Can you work these out from the model? Positions are in its coordinate system, mm. Face numbers are marked on the shaded views. A direction names the side the tool comes from. Coordinates: 2 decimals unless noted, no trailing zeros. Order: outer loops, then holes, each group sorted by start corner. A loop starts at its lowest first (then second) coordinate and runs counter-clockwise, first axis right, second up.
Autodesk Inventor part; units mm, degrees
ref_plane "YZ Plane" through (0, 0, 0) normal (1, 0, 0) x (0, 1, 0)
ref_plane "XZ Plane" through (0, 0, 0) normal (0, 1, 0) x (-1, 0, 0)
ref_plane "XY Plane" through (0, 0, 0) normal (0, 0, 1) x (1, 0, 0)
sketch "Sketch1" plane through (0, 0, 0) normal (0, 0, 1) x (1, 0, 0)
  line L0 (0, 0) -> (152.4, 0)
  line L1 (152.4, 0) -> (152.4, 101.6)
  line L2 (152.4, 101.6) -> (0, 101.6)
  line L3 (0, 101.6) -> (0, 0)
  line L4 (0, 0) -> (12.7, 0)
  line L5 (12.7, 0) -> (12.7, 12.7)
  line L6 (12.7, 12.7) -> (139.7, 12.7)
  line L7 (139.7, 12.7) -> (139.7, 88.9)
  line L8 (139.7, 88.9) -> (12.7, 88.9)
  line L9 (12.7, 88.9) -> (12.7, 12.7)
  line L10 (69.85, 101.6) -> (82.55, 101.6)
  line L11 (82.55, 101.6) -> (82.55, 0)
  line L12 (82.55, 0) -> (69.85, 0)
  line L13 (69.85, 0) -> (69.85, 101.6)
  line L14 (69.85, 101.6) -> (82.55, 0) construction
  line L15 (82.55, 101.6) -> (69.85, 0) construction
  point P0 (76.2, 50.8)
  point P1 (82.55, 88.9)
  point P2 (82.55, 12.7)
  point P3 (69.85, 12.7)
  point P4 (69.85, 88.9)
  dimension "d0" = 152.4
  dimension "d1" = 101.6
  dimension "d2" = 12.7
  dimension "d3" = 12.7
  dimension "d4" = 127
  dimension "d5" = 76.2
  dimension "d6" = 12.7
extrude "Extrusion1" add sketch "Sketch1" along normal blind 12.7 contours L3 L2 L13 L8 L9 L5 L0 | L5 L6 L13 L0 | L13 L6 L11 L0 | L2 L11 L8 L13 | L11 L6 L7 L8 L2 L1 L0 | L13 L8 L11 L6
sketch "Sketch2" plane through (0, 101.6, 0) normal (0, 1, 0) x (1, 0, 0)
  line L0 (69.85, 0) -> (69.85, -12.7)
  line L1 (82.55, 0) -> (82.55, -12.7)
  line L2 (139.7, 0) -> (139.7, -12.7)
  line L3 (12.7, 0) -> (12.7, -12.7)
  line L4 (12.7, 0) -> (12.7, -12.7)
  line L5 (12.7, -6.35) -> (63.5, -6.35)
  line L6 (69.85, -6.35) -> (76.2, -6.35)
  point P0 (0, 0)
  dimension "d9" = 50.8
  dimension "d17" = 6.35
sketch "Sketch4" plane through (69.85, 12.7, 0) normal (1, 0, 0) x (0, 0, -1)
  line L0 (0, 76.2) -> (-12.7, 76.2)
  line L1 (-6.35, 76.2) -> (-6.35, 50.8)
  line L2 (-6.35, 76.2) -> (19.05, 76.2) construction
  line L3 (-6.35, 50.8) -> (-6.35, 25.4)
  line L4 (0, 0) -> (0, 76.2)
  line L5 (-12.7, 52.3875) -> (0, 52.3875)
  line L6 (0, 52.3875) -> (0, 49.2125)
  line L7 (0, 49.2125) -> (-12.7, 49.2125)
  line L8 (-12.7, 49.2125) -> (-12.7, 52.3875)
  line L9 (-12.7, 52.3875) -> (0, 49.2125) construction
  line L10 (0, 52.3875) -> (-12.7, 49.2125) construction
  line L11 (-12.7, 23.8125) -> (0, 23.8125)
  line L12 (0, 23.8125) -> (0, 26.9875)
  line L13 (0, 26.9875) -> (-12.7, 26.9875)
  line L14 (-12.7, 26.9875) -> (-12.7, 23.8125)
  line L15 (-12.7, 23.8125) -> (0, 26.9875) construction
  line L16 (0, 23.8125) -> (-12.7, 26.9875) construction
  point P0 (0, -12.7)
  dimension "d25" = 25.4
  dimension "d26" = 90
  dimension "d27" = 25.4
  dimension "d28" = 180
  dimension "d29" = 3.175
  dimension "d30" = 3.175
extrude "Extrusion2" add sketch "Sketch4" against normal blind 12.7 contours L4 L7 L3 L1 L5 | L1 L3 L7 L8 L5 | L4 L11 L14 L13
hole "Hole1" at (63.5, 101.6, 6.35) direction (0, -1, 0) diameter 1.8415 end through all both
hole "Hole2" at (63.5, 101.6, 6.35) direction (0, -1, 0) diameter 3.429 depth 3.175
ref_plane "Work Plane1" through (76.2, 101.6, 6.35) normal (1, 0, 0) x (0, 0, -1)
ref_plane "Work Plane2" through (76.2, 50.8, 0) normal (0, 1, 0) x (1, 0, 0)
mirror "Mirror1" about plane through (76.2, 101.6, 6.35) normal (1, 0, 0) of "Hole1", "Hole2", "Extrusion2"
mirror "Mirror2" about plane through (76.2, 50.8, 0) normal (0, 1, 0) of "Hole1", "Hole2", "Mirror1"
sketch "Sketch5" plane through (0, 0, 0) normal (-1, 0, 0) x (0, 0, 1)
  line L0 (12.7, 61.9125) -> (12.7, 39.6875)
  line L1 (12.7, 50.8) -> (12.7, 76.2)
  line L2 (12.7, 76.2) -> (0, 76.2)
  line L3 (0, 76.2) -> (0, 25.4)
  line L4 (0, 25.4) -> (12.7, 25.4)
  line L5 (12.7, 25.4) -> (12.7, 76.2)
  line L6 (4.6355, 101.6) -> (8.0645, 101.6)
  line L7 (6.35, 101.6) -> (6.35, 76.2)
  line L8 (6.35, 76.2) -> (6.35, 25.4)
  line L9 (0, 12.7) -> (12.7, 12.7)
  line L10 (0, 88.9) -> (0, 12.7)
  line L11 (12.7, 76.2) -> (0, 76.2)
  line L12 (0, 76.2) -> (0, 79.375)
  line L13 (0, 79.375) -> (12.7, 79.375)
  line L14 (12.7, 79.375) -> (12.7, 76.2)
  line L15 (0, 101.6) -> (12.7, 101.6)
  line L16 (0, 101.6) -> (0, 0)
  line L17 (12.7, 101.6) -> (0, 101.6)
  line L18 (0, 101.6) -> (0, 98.425)
  line L19 (0, 98.425) -> (12.7, 98.425)
  line L20 (12.7, 98.425) -> (12.7, 101.6)
  dimension "d33" = 25.4
  dimension "d34" = 50.8
  dimension "d35" = 25.4
  dimension "d36" = 50.8
  dimension "d37" = 180
  dimension "d45" = 3.175
  dimension "d62" = 3.175
hole "Hole3" [suppressed]
extrude "Extrusion3" cut sketch "Sketch5" against normal blind 12.7 contours L0 L5 L4 L8 L2 L1 | L8 L4 L3 L2
extrude "Extrusion4" add sketch "Sketch5" along normal blind 28.575 contours L19 L16 L15 L6 L7 | L7 L6 L15 L20 L19
sketch "Sketch6" plane through (12.7, 98.425, 0) normal (0, -1, 0) x (1, 0, 0)
  line L0 (-12.7, 12.7) -> (0, 12.7)
  line L1 (0, 0) -> (-12.7, 0)
  line L2 (-41.275, 12.7) -> (-38.1, 12.7)
  line L3 (-38.1, 12.7) -> (-38.1, 0)
  line L4 (-38.1, 0) -> (-41.275, 0)
  line L5 (-41.275, 0) -> (-41.275, 12.7)
  dimension "d50" = 3.175
extrude "Extrusion5" add sketch "Sketch6" along normal blind 57.15
sketch "Sketch7" plane through (-28.575, 0, 0) normal (-1, 0, 0) x (0, 0, 1)
  line L0 (12.7, 88.9) -> (12.7, 12.7)
  line L1 (12.7, 38.0513) -> (6.35, 38.0513)
  line L2 (5.4292, 36.5125) -> (5.4292, 39.6875)
  line L3 (6.35, 38.0513) -> (6.35, 50.7513)
  point P0 (0, 0)
  dimension "d53" = 6.35
  dimension "d54" = 12.7
hole "Hole4" at (-28.575, 50.7513, 6.35) direction (1, 0, 0) diameter 6.7564 depth 25.4
mirror "Mirror3" about plane through (76.2, 101.6, 6.35) normal (1, 0, 0) of "Extrusion3", "Extrusion4", "Extrusion5", "Hole4"
sketch "Sketch8" plane through (69.85, 88.9, 0) normal (-1, 0, 0) x (0, 0, 1)
  line L0 (12.7, 0) -> (12.7, -23.8125)
  line L1 (12.7, 0) -> (6.35, 0)
  line L2 (12.7, 0) -> (19.05, 0) construction
  line L3 (6.35, 0) -> (6.35, -12.7)
  point P0 (0, -88.9)
  dimension "d63" = 6.35
  dimension "d64" = 180
  dimension "d65" = 12.7
hole "Hole5" at (69.85, 76.2, 6.35) direction (1, 0, 0) diameter 6.7564 depth 25.4 counterbore diameter 11.1252 counterbore depth 6.35
ref_plane "Work Plane3" through (82.55, 101.6, 6.35) normal (1, 0, 0) x (0, 0, -1)
split "Split1" plane through (82.55, 101.6, 6.35) removes the side toward (1, 0, 0)
mirror "Mirror4" about plane through (76.2, 50.8, 0) normal (0, 1, 0) of "Hole5"
properties part number "SampleHolder"
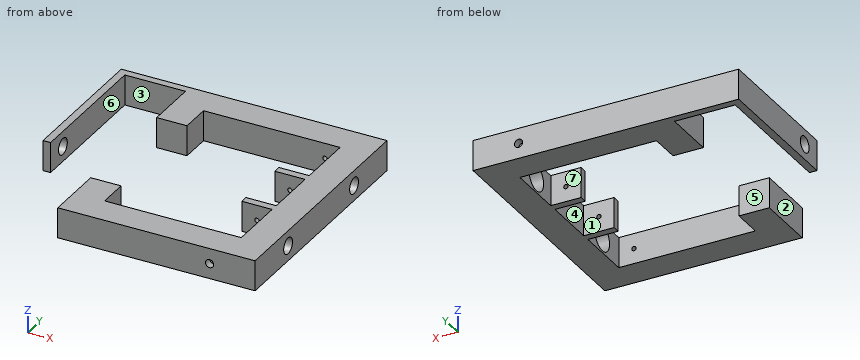
1. Thinking about a two-plate mould opening in X: for the marked faces 1, 2, 3 and 4, which applies, pulls with the +X half, pulls with the -X half, needs draft (parallel to the pull), parting line crosses it, or undercut?
Completed:
face 1: needs draft
face 2: pulls with the -X half
face 3: undercut
face 4: undercut
2. Imagine slicing it at C-C on x = -18. Please give me the cut outline in (y, z) (3 decimals).
Completed:
outline: (98.425, 0) - (101.6, 0) - (101.6, 12.7) - (98.425, 12.7) - close
3. I'm going to push flat-ended pins straight in: pin 1 (2.5 mm diameter, centred on x = 63.5, z = 6.35, fed in from -Y) (3 decimals); pin 2 (1.6 mm diameter, centred on x = -27.5, z = 7.5, fed in from -Y) (3 decimals); pin 3 (5 mm diameter, centred on x = 18.5, z = 1.5, fed in from -Y); pin 4 (1 mm diameter, centred on x = -13.5, z = 7.5, fed in from -Y) (3 decimals). Where does each tip first touch, or does it pass through?
Completed:
pin 1: stops at y = 3.175
pin 2: stops at y = 41.275
pin 3: stops at y = 0
pin 4: stops at y = 98.425
4. Imagine slicing it at A-A on x = 59. Please give me the cut outline in (y, z), then the cut area to 3 significant figures.
Completed:
outline: (0, 0) - (12.7, 0) - (12.7, 12.7) - (0, 12.7) - close; (36.51, 0) - (39.69, 0) - (39.69, 12.7) - (36.51, 12.7) - close; (61.91, 0) - (65.09, 0) - (65.09, 12.7) - (61.91, 12.7) - close; (88.9, 0) - (101.6, 0) - (101.6, 12.7) - (88.9, 12.7) - close
area: 403 mm2
5. Imagine slicing it at B-B on y = 10. Please give me the cut outline in (x, z), then the cut area to 3 significant figures.
Completed:
outline: (0, 0) - (82.55, 0) - (82.55, 12.7) - (0, 12.7) - close; hole circle Ø1.84 at (63.5, 6.35)
area: 1,050 mm2
6. Please list where these lines run through material, in increasing order: probe 1 along X at (y, z) = (63.2, 6.35) (3 decimals); probe 2 along X at (y, z) = (80.5, 1.5) (3 decimals); probe 3 along Z at (x, y) = (78.5, 25.4).
Completed:
probe 1: x = -28.575 to -25.4, 57.15 to 62.579, 64.421 to 82.55
probe 2: x = -28.575 to -25.4, 0 to 12.7, 69.85 to 82.55
probe 3: z = 0 to 2.97, 9.73 to 12.7
7. On a 3-axis mill with a long thin cutter (end or side, diameter ignored), from which of +Z, -Z, +X, -X, +Y, -Y can I reach the whole of each face in a straight line? I mean the marked faces 5, 6 and 7. Say none if no direction works.
Completed:
face 5: +Z, -Z, -X
face 6: +Z, -Z, -Y
face 7: +Z, -Z
